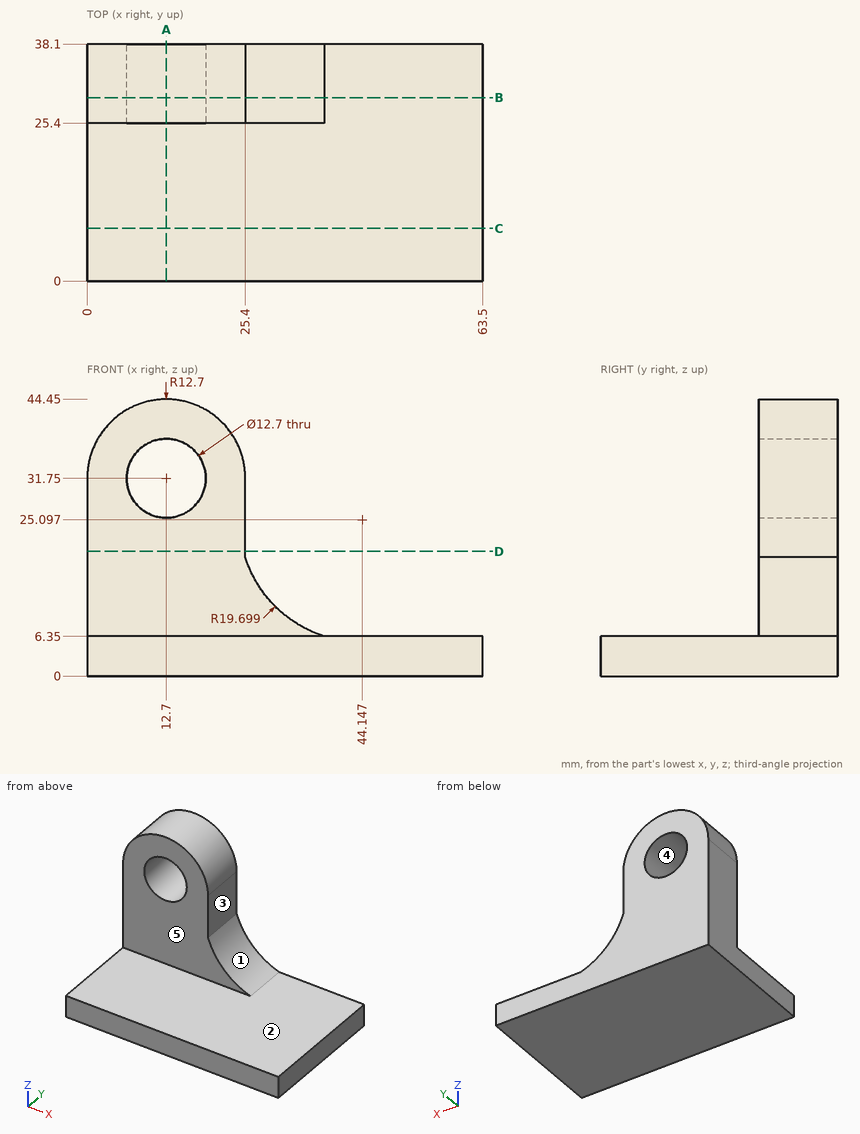
Print and shaded views of the part. All mm, measured from the part's lowest x, y and z. A direction names the side the tool comes from. Coordinates: 2 decimals unless noted, no trailing zeros. Order: outer loops, then holes, each group sorted by start corner. A loop starts at its lowest first (then second) coordinate and runs counter-clockwise, first axis right, second up. Notation, with made-up numbers: (71, 71) -> (84, 71) arc R21 ccw to (84, 101) -> close; hole circle Ø2 at (-13, -14.75). An arc over 180 degrees is marked (long way). Use one line per item in the form item = value. Start each with the question number.
1) Tool access for the marked faces 1 and 2: list every direction of +Z, -Z, +X, -X, +Y, -Y with a clear straight run to the whole face (end or side of a thin tool).
2) Pull direction X, two halves, no side cores. Call the marked faces 3, 4 and 5: +X half, -X half, draft (parallel to the pull), parting line (faces both ways), or undercut.
3) Band-saw the part on D-D on z = 20. Give the cut face in (x, y).
4) Band-saw the part on B-B on y = 29.5. Give the cut face in (x, z), then the cut area to 3 significant figures.
5) Drill centre lines: L1, parallel to Z at x = 60, y = 26.5; L2, parallel to Z at x = 12.7, y = 33; L3, parallel to Y at x = 19, z = 11. Where is each one in solid material? Low to high. Write a range as [from, to].
6) Band-saw the part on A-A on x = 12.7. Give the cut face in (y, z).
7) Band-saw the part on C-C on y = 8.5. Give the cut face in (x, z), then the cut area to 3 significant figures.
8) Drop flat-ended pins along their axis: pin 1 (10 mm diameter, centred on x = 10.5, z = 17, fed in from -Y); pin 2 (10 mm diameter, centred on y = 29.5, z = 25, fed in from +X); pin 3 (3 mm diameter, centred on x = 34, y = 4, fed in from +Z). Give the stop position or say it passes through.
Entries:
q1.face_1 = +Z, +X, +Y, -Y
q1.face_2 = +Z, +X, -Y
q2.face_3 = +X half
q2.face_4 = undercut
q2.face_5 = draft
q3.outline = (0, 25.4) -> (25.4, 25.4) -> (25.4, 38.1) -> (0, 38.1) -> close
q4.outline = (0, 0) -> (63.5, 0) -> (63.5, 6.35) -> (38.1, 6.35) arc R19.7 cw to (25.4, 19.05) -> (25.4, 31.75) arc R12.7 ccw to (0, 31.75) -> close; hole circle Ø12.7 at (12.7, 31.75)
q4.area = 1,230 mm2
q5.L1 = [0, 6.35]
q5.L2 = [0, 25.4], [38.1, 44.45]
q5.L3 = [25.4, 38.1]
q6.outline = (0, 0) -> (38.1, 0) -> (38.1, 25.4) -> (25.4, 25.4) -> (25.4, 6.35) -> (0, 6.35) -> close; (25.4, 38.1) -> (38.1, 38.1) -> (38.1, 44.45) -> (25.4, 44.45) -> close
q7.outline = (0, 0) -> (63.5, 0) -> (63.5, 6.35) -> (0, 6.35) -> close
q7.area = 403 mm2
q8.pin_1 = 25.4
q8.pin_2 = 25.4
q8.pin_3 = 6.35
